Verification items for the finished model (mm, model axes). Face numbers are marked on the shaded views. A direction names the side the tool comes from. Give positions to 0.01 mm unless a question says otherwise; leave off trailing zeros. Loops run counter-clockwise (first coordinate to the right, second up) from the corner with the lowest first, then second, coordinate; pieces in that order, holes last. Notation, with made-up numbers: (75, -32) - (119, -32) arc R25 cw to (119, -15) - close; hole circle Ø1 at (40.5, 10.25). An arc over 180 degrees is marked (long way). Answer in a Markdown table with one row per item.
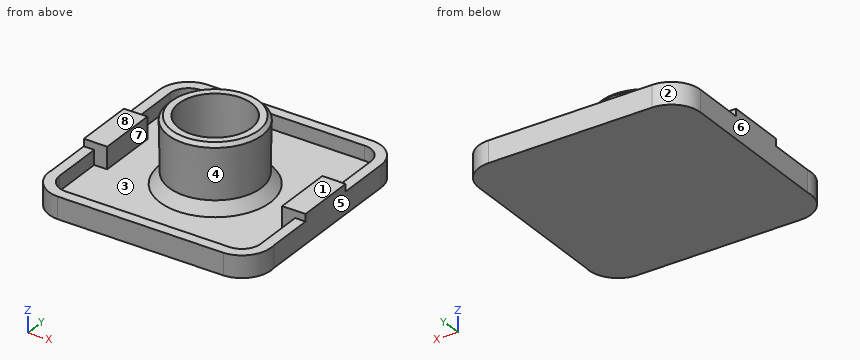
```python
from build123d import *

# Parameters (mm, degrees)
EXTRUDE_1_DEPTH     = 1
EXTRUDE_2_DEPTH     = 3
SKETCH_1_4_R        = 6.3
EXTRUDE_3_DEPTH     = 10
EXTRUDE_3_DRAFT     = -1
SKETCH_1_5_W        = 1.42302488
SKETCH_1_5_H        = 8.2
SKETCH_1_5_W_2      = 1.791144373
EXTRUDE_4_DEPTH     = 4
CHAMFER_1_SIZE      = 0.5
CHAMFER_1_SIZE2     = 0.491497051
SKETCH_2_R          = 5
CUT_EXTRUDE_1_DEPTH = 9
CHAMFER_2_SIZE      = 1.5
CHAMFER_2_SIZE_2    = 1.284636358
CHAMFER_2_SIZE_3    = 1.303930107


# Read off the part's stored shape, not the designer's step: Бобышка-Вытянуть1
with BuildPart() as part:
    # Бобышка-Вытянуть1 outline → Бобышка-Вытянуть1 (new body)
    with BuildSketch(Plane.XY):
        with BuildLine():
            Line((-15.25, 11.25), (-15.25, -10.65))
            ThreePointArc((-15.25, -10.65), (-14.365417418, -13.829568629), (-11.406655615, -15.291714861))
            Line((-11.406655615, -15.291714861), (11.406655615, -15.291714861))
            ThreePointArc((11.406655615, -15.291714861), (14.365417418, -13.829568629), (15.25, -10.65))
            Line((15.25, -10.65), (15.25, 11.25))
            ThreePointArc((15.25, 11.25), (14.078427125, 14.078427125), (11.25, 15.25))
            Line((11.25, 15.25), (-11.25, 15.25))
            ThreePointArc((-11.25, 15.25), (-14.078427125, 14.078427125), (-15.25, 11.25))
        make_face()
    extrude(amount=EXTRUDE_1_DEPTH)

    # Эскиз1<3> → Бобышка-Вытянуть2 (add)
    with BuildSketch(Plane.XY):
        with BuildLine():
            ThreePointArc((-11.25, 15.25), (-14.078427125, 14.078427125), (-15.25, 11.25))
            Line((-15.25, 11.25), (-15.25, -10.65))
            ThreePointArc((-15.25, -10.65), (-14.365417418, -13.829568629), (-11.406655615, -15.291714861))
            Line((-11.406655615, -15.291714861), (11.406655615, -15.291714861))
            ThreePointArc((11.406655615, -15.291714861), (14.365417418, -13.829568629), (15.25, -10.65))
            Line((15.25, -10.65), (15.25, 11.25))
            ThreePointArc((15.25, 11.25), (14.078427125, 14.078427125), (11.25, 15.25))
            Line((11.25, 15.25), (-11.25, 15.25))
        make_face()
        with BuildLine():
            ThreePointArc((13.82697512, -11.25), (13.072196582, -13.072196582), (11.25, -13.82697512))
            Line((11.25, -13.82697512), (-11.25, -13.82697512))
            ThreePointArc((-11.25, -13.82697512), (-13.072196582, -13.072196582), (-13.82697512, -11.25))
            Line((-13.82697512, -11.25), (-13.82697512, -4.195156857))
            Line((-13.82697512, -4.195156857), (-12.035830747, -4.195156857))
            Line((-12.035830747, -4.195156857), (-12.035830747, 4.004843143))
            Line((-12.035830747, 4.004843143), (-13.82697512, 4.004843143))
            Line((-13.82697512, 4.004843143), (-13.82697512, 11.25))
            ThreePointArc((-13.82697512, 11.25), (-13.072196582, 13.072196582), (-11.25, 13.82697512))
            Line((-11.25, 13.82697512), (11.25, 13.82697512))
            ThreePointArc((11.25, 13.82697512), (13.072196582, 13.072196582), (13.82697512, 11.25))
            Line((13.82697512, 11.25), (13.82697512, 4.004843143))
            Line((13.82697512, 4.004843143), (12.035830747, 4.004843143))
            Line((12.035830747, 4.004843143), (12.035830747, -4.195156857))
            Line((12.035830747, -4.195156857), (13.82697512, -4.195156857))
            Line((13.82697512, -4.195156857), (13.82697512, -11.25))
        make_face(mode=Mode.SUBTRACT)
    extrude(amount=EXTRUDE_2_DEPTH)


with BuildPart() as extrude_3_tool:
    # Эскиз1<4> → Бобышка-Вытянуть3 (with draft: the straight prism first)
    with BuildSketch(Plane.XY):
        Circle(SKETCH_1_4_R)
    extrude(amount=EXTRUDE_3_DEPTH)
    # Бобышка-Вытянуть3: the draft: its side faces are tilted about the plane it starts from
    extrude_3_sides = [extrude_3_tool.faces().sort_by_distance(p)[0] for p in [
        (-6.3, 0, 5),
    ]]
    draft(extrude_3_sides, Plane.XY, EXTRUDE_3_DRAFT)


with BuildPart() as part_1:
    add(part.part)

    # Бобышка-Вытянуть3: add extrude_3_tool
    add(extrude_3_tool.part)

    # Эскиз1<5> → Бобышка-Вытянуть4 (add)
    with BuildSketch(Plane.XY):
        with Locations((-14.53848756, -0.095156857)):
            Rectangle(SKETCH_1_5_W, SKETCH_1_5_H)
        with Locations((-12.931402933, -0.095156857)):
            Rectangle(SKETCH_1_5_W_2, SKETCH_1_5_H)
        with Locations((12.931402933, -0.095156857)):
            Rectangle(SKETCH_1_5_W_2, SKETCH_1_5_H)
        with Locations((14.53848756, -0.095156857)):
            Rectangle(SKETCH_1_5_W, SKETCH_1_5_H)
    extrude(amount=EXTRUDE_4_DEPTH)

    # Фаска1
    chamfer_1_edges = [part_1.edges().sort_by_distance(p)[0] for p in [
        (-6.474550649, 0, 10),
    ]]
    chamfer_1_side = [part_1.faces().sort_by_distance(p)[0] for p in [
        (-6.396002857, 0, 5.5),
    ]]
    chamfer(chamfer_1_edges, length=CHAMFER_1_SIZE, length2=CHAMFER_1_SIZE2, reference=chamfer_1_side[0])

    # Эскиз2 → Вырез-Вытянуть1 (cut)
    with BuildSketch(Plane.XY.offset(10)):
        Circle(SKETCH_2_R)
    extrude(amount=-CUT_EXTRUDE_1_DEPTH, mode=Mode.SUBTRACT)

    # Фаска2
    # the kernel refuses this chamfer: 1.5, 1.303930107, 1.284636358 mm, written as the material it adds along each edge
    with BuildSketch(Plane(origin=(0, 0, 1), x_dir=(1, 0, 0), z_dir=(0, 1, 0))) as chamfer_2_piece_1:
        Polygon((6.317455065 + CHAMFER_2_SIZE * 0.0174524064373, -CHAMFER_2_SIZE * 0.999847695156), (6.317455065 + CHAMFER_2_SIZE_2, 0), (6.317455065, 0), align=None)
    revolve(axis=Axis((0, 0, 1), (0, 0, -1)))
    with BuildSketch(Plane(origin=(0, 0, 1), x_dir=(1, 0, 0), z_dir=(0, -1, 0))) as chamfer_2_piece_2:
        Polygon((5, CHAMFER_2_SIZE), (5 - CHAMFER_2_SIZE_3, 0), (5, 0), align=None)
    revolve(axis=Axis((0, 0, 1), (0, 0, 1)))


solid = part_1.part
```
Q1. Sectioned sample at C-C (z = 7.75). Record the cut outline in (x, y).
Completed:
| item | result |
|---|---|
| outline | circle Ø12.87 at (0, 0); hole circle Ø10 at (0, 0) |
Q2. Sectioned sample at B-B (y = 12). Record the cut outline in (x, z).
Completed:
| item | result |
|---|---|
| outline | (-15.18, 0) - (15.18, 0) - (15.18, 3) - (13.72, 3) - (13.72, 1) - (-13.72, 1) - (-13.72, 3) - (-15.18, 3) - close |
Q3. Draft check along X on the marked faces 1, 2, 3 and 4. Enter one of: +X half, -X half, draft (parallel to the pull), parting line (faces both ways), or undercut.
Completed:
| item | result |
|---|---|
| face 1 | draft |
| face 2 | -X half |
| face 3 | undercut |
| face 4 | undercut |
Q4. Sectioned sample at A-A (x = -10). Record the cut outline in (y, z), and give its area (3 significant figures).
Completed:
| item | result |
|---|---|
| outline | (-15.29, 0) - (15.25, 0) - (15.25, 3) - (13.83, 3) - (13.83, 1) - (-13.83, 1) - (-13.83, 3) - (-15.29, 3) - close |
| area | 36.3 mm^2 |
Q5. Thickness scan on line 1 (Z direction, x = -7, y = -8); line 2 (Y direction, x = 4.5, z = 7.25); line 3 (Y direction, x = 0, z = 6.75). Record the ranges inside material, lowest first.
Completed:
| item | result |
|---|---|
| line 1 | 0 to 1 |
| line 2 | -4.59 to -2.18, 2.18 to 4.59 |
| line 3 | -6.42 to -5, 5 to 6.42 |
Q6. Tool access check on the marked faces 5, 6, 7 and 8. Record the directions out of +Z, -Z, +X, -X, +Y, -Y that give a thin tool (end or side, any length) a straight path to the whole face; none if there is none.
Completed:
| item | result |
|---|---|
| face 5 | +Z, -Z, +X, +Y |
| face 6 | +Z, -Z, -X, +Y |
| face 7 | +Z |
| face 8 | +Z, -X, +Y, -Y |
Q7. Sectioned sample at D-D (x = 12.5). Record the cut outline in (y, z).
Completed:
| item | result |
|---|---|
| outline | (-15.1, 0) - (15.05, 0) - (15.05, 3) - (13.5, 3) - (13.5, 1) - (4, 1) - (4, 4) - (-4.2, 4) - (-4.2, 1) - (-13.5, 1) - (-13.5, 3) - (-15.1, 3) - close |
Q8. Go/stop test with flat-tipped pins: P1, Ø3.5, axis at x = 13.5, z = 3, coming from the +Y side; P2, Ø2, axis at y = -2.5, z = 8.5, coming from the +X side; P3, Ø5, axis at y = 8, z = 1, coming from the +X side. Record where each tip stops, or that it passes through.
Completed:
| item | result |
|---|---|
| P1 | y = 15.22 |
| P2 | x = 6.27 |
| P3 | x = 15.25 |
